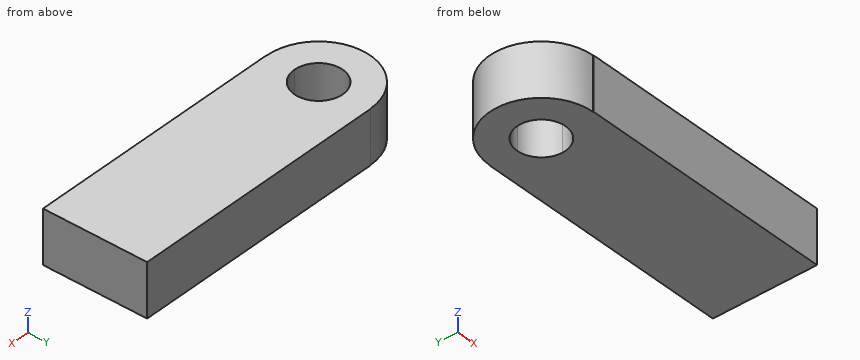
from build123d import *

# Parameters (mm, degrees)
F1_DEPTH = 25.4


with BuildPart() as f1:
    # F0 (on Top) → F1 (new body)
    with BuildSketch(Plane.XY):
        with BuildLine():
            Line((-61.765037477, -24.7485272537), (-61.765037477, -24.9177198857))
            Line((-61.765037477, -24.9177198857), (61.765037477, -24.9177198857))
            Line((61.765037477, -24.9177198857), (61.765037477, 24.9177198857))
            Line((61.765037477, 24.9177198857), (-61.765037477, 24.9177198857))
            Line((-61.765037477, 24.9177198857), (-61.765037477, 24.7485272537))
            ThreePointArc((-61.765037477, 24.7485272537), (-44.2651860316, 17.4998514455), (-37.0165102233, 0))
            ThreePointArc((-37.0165102233, 0), (-44.2651860316, -17.4998514455), (-61.765037477, -24.7485272537))
        make_face()
        with BuildLine():
            ThreePointArc((-61.765037477, 24.7485272537), (-86.5135647307, 0), (-61.765037477, -24.7485272537))
            Line((-61.765037477, -24.7485272537), (-61.765037477, -11.5415442381))
            ThreePointArc((-61.765037477, -11.5415442381), (-73.3065817151, 0), (-61.765037477, 11.5415442381))
            Line((-61.765037477, 11.5415442381), (-61.765037477, 24.7485272537))
        make_face()
        with BuildLine():
            Line((-61.765037477, -11.5415442381), (-61.765037477, -24.7485272537))
            ThreePointArc((-61.765037477, -24.7485272537), (-44.2651860316, -17.4998514455), (-37.0165102233, 0))
            ThreePointArc((-37.0165102233, 0), (-44.2651860316, 17.4998514455), (-61.765037477, 24.7485272537))
            Line((-61.765037477, 24.7485272537), (-61.765037477, 11.5415442381))
            ThreePointArc((-61.765037477, 11.5415442381), (-53.6039332809, 8.1611041961), (-50.2234932389, 0))
            ThreePointArc((-50.2234932389, 0), (-53.6039332809, -8.1611041961), (-61.765037477, -11.5415442381))
        make_face()
    extrude(amount=F1_DEPTH)


solid = f1.part
Verification items for the finished model (mm, model axes). Coordinates: 2 decimals unless noted, no trailing zeros. Order: outer loops, then holes, each group sorted by start corner. A loop starts at its lowest first (then second) coordinate and runs counter-clockwise, first axis right, second up. Notation, with made-up numbers: (67, 72) -> (110, 72) arc R13 cw to (110, 84) -> close; hole circle Ø3 at (-19.75, 86.25). An arc over 180 degrees is marked (long way). Put each result on its own line as item: value. Start each with the question number.
1. Cross-section at A-A, the plane z = 10.75. Record the boundary of the cut face in (x, y).
2. Cross-section at B-B, the plane x = -58. Record the boundary of the cut face in (y, z), then the cut area to 3 significant figures.
3. Cross-section at C-C, the plane y = 2. Record the boundary of the cut face in (x, z).
4. Go/stop test with flat-tipped pins: pin 1 Ø6 at (y, z) = (-16, 12) entering from -X; pin 2 Ø4 at (y, z) = (18.5, 15.5) entering from -X; pin 3 Ø1 at (y, z) = (14, 12) entering from -X. Record where each tip stops, or that it passes through.
5. Material ranges on L1, parallel to Y at x = -61, z = 2.25; L2, parallel to X at y = -7.5, z = 10.25; L3, parallel to Y at x = -63.5, z = 18, recorded low to high. Write a range as [from, to].
6. Cross-section at D-D, the plane y = -15. Record the boundary of the cut face in (x, z), then the cut area to 3 significant figures.
Computed:
1. outline: (-61.77, -24.92) -> (61.77, -24.92) -> (61.77, 24.92) -> (-61.77, 24.92) -> (-61.77, 24.75) arc R24.75 ccw to (-61.77, -24.75) -> close; hole circle Ø23.08 at (-61.77, 0)
2. outline: (-24.92, 0) -> (-10.91, 0) -> (-10.91, 25.4) -> (-24.92, 25.4) -> close; (10.91, 0) -> (24.92, 0) -> (24.92, 25.4) -> (10.91, 25.4) -> close
2. area: 712 mm2
3. outline: (-86.43, 0) -> (-73.13, 0) -> (-73.13, 25.4) -> (-86.43, 25.4) -> close; (-50.4, 0) -> (61.77, 0) -> (61.77, 25.4) -> (-50.4, 25.4) -> close
4. pin 1: x = -82.82
4. pin 2: x = -80.21
4. pin 3: x = -82.51
5. L1: [-24.92, -11.52], [11.52, 24.92]
5. L2: [-85.35, -70.54], [-52.99, 61.77]
5. L3: [-24.69, -11.41], [11.41, 24.69]
6. outline: (-81.45, 0) -> (61.77, 0) -> (61.77, 25.4) -> (-81.45, 25.4) -> close
6. area: 3,640 mm2
